```python
from build123d import *

# Parameters (mm, degrees)
SKETCH1_R                = 6
SKETCH1_R_2              = 4
BOSS_EXTRUDE1_DEPTH      = 4
BOSS_EXTRUDE2_DEPTH      = 2
BOSS_EXTRUDE2_DEPTH_BACK = 1
SKETCH2_R                = 1.5
CUT_EXTRUDE1_DEPTH       = 1.5


with BuildPart() as part:
    # Sketch1 → Boss-Extrude1 (new body)
    with BuildSketch(Plane.XY):
        Circle(SKETCH1_R)
        Circle(SKETCH1_R_2, mode=Mode.SUBTRACT)
    extrude(amount=BOSS_EXTRUDE1_DEPTH)

    # Sketch2 → Boss-Extrude2 (add, two sides: drawn at the far end of the back side and taken through both)
    with BuildSketch(Plane(origin=(6, 0, 0), x_dir=(0, 0, -1), z_dir=(1, 0, 0)).offset(-BOSS_EXTRUDE2_DEPTH_BACK)):
        with Locations((-2, 0)):
            Circle(SKETCH2_R)
    extrude(amount=BOSS_EXTRUDE2_DEPTH + BOSS_EXTRUDE2_DEPTH_BACK)

    # Sketch3 → Cut-Extrude1 (cut)
    with BuildSketch(Plane(origin=(8, 0, 0), x_dir=(0, 0, -1), z_dir=(1, 0, 0))):
        Polygon((-2.490747729, 0.85), (-1.509252271, 0.85), (-1.018504542, 0), (-1.509252271, -0.85), (-2.490747729, -0.85), (-2.981495458, 0), align=None)
    extrude(amount=-CUT_EXTRUDE1_DEPTH, mode=Mode.SUBTRACT)


solid = part.part
```
Design review of the part built by this model. Coordinates are the model's own, in mm. A direction names the side the tool comes from. Give positions to 0.01 mm unless a question says otherwise; leave off trailing zeros. Write each loop counter-clockwise with the first axis right and the second up, starting at its lowest first coordinate (ties: lowest second). Pieces come first, ordered by that corner, then holes.
(1) Add section D-D (y = -0.25). Give the boundary of the cut face in (x, z).
Checked values:
outline: (-5.99, 0) - (-3.99, 0) - (-3.99, 4) - (-5.99, 4) - close; (3.99, 0) - (5.99, 0) - (5.99, 0.52) - (8, 0.52) - (8, 1.16) - (6.5, 1.16) - (6.5, 2.84) - (8, 2.84) - (8, 3.48) - (5.99, 3.48) - (5.99, 4) - (3.99, 4) - close
(2) Add section B-B (y = -3.5). Give the boundary of the cut face in (x, z), and give its area (3 significant figures).
Checked values:
outline: (-4.87, 0) - (-1.94, 0) - (-1.94, 4) - (-4.87, 4) - close; (1.94, 0) - (4.87, 0) - (4.87, 4) - (1.94, 4) - close
area: 23.5 mm2
(3) Mouldability with a two-part tool opening along X and no side actions: class faces 3 (the face through (8, -1, 2)), 4 (the face through (-1.42, -3.92, 0)), 5 (the face through (-0.867, -3.905, 1.972)) as +X half, -X half, draft (parallel to the pull), parting line (faces both ways), or undercut.
Checked values:
face 3: +X half
face 4: draft
face 5: undercut
(4) Tool access review of faces 1 (the face through (7.26, 0.42, 2.74)), 2 (the face through (-1.42, -3.92, 4)): name each direction out of +Z, -Z, +X, -X, +Y, -Y from which nothing blocks a thin tool from reaching the whole face with its end or side.
Checked values:
face 1: +X
face 2: +Z, +X, -X, +Y, -Y
(5) Clearance check with flat-ended pins moving along their axes: pin 1 Ø2 at (x, z) = (-1.5, 1.5) entering from -Y; pin 2 Ø1.1 at (x, z) = (7, 2) entering from -Y; pin 3 Ø2 at (y, z) = (-4, 2.5) entering from -X. State where each tip first meets the part, or that it passes through.
Checked values:
pin 1: stops at y = -5.98
pin 2: stops at y = -1.5
pin 3: stops at x = -5.2
(6) Add section C-C (z = 3.25). Give the boundary of the cut face in (x, y), and give its area (3 significant figures).
Checked values:
outline: (5.94, -0.83) - (8, -0.83) - (8, 0.83) - (5.94, 0.83) arc R6 ccw (long way) to start; hole circle Ø8 at (0, 0)
area: 66.2 mm2
(7) Wall thickness on line 1 along Y through (x, z) = (0, 0.95); line 2 along X through (y, z) = (-0.75, 2.9); line 3 along X through (y, z) = (2.5, 0.55): over which ranges is each line inside the solid? List them lowest first.
Checked values:
line 1: y = -6 to -4, 4 to 6
line 2: x = -5.95 to -3.93, 3.93 to 8
line 3: x = -5.45 to -3.12, 3.12 to 5.45
(8) Add section A-A (x = 0). Give the boundary of the cut face in (y, z).
Checked values:
outline: (-6, 0) - (-4, 0) - (-4, 4) - (-6, 4) - close; (4, 0) - (6, 0) - (6, 4) - (4, 4) - close
